Here's how the part is built. I have some questions about the finished solid (model axes, mm). Face numbers are marked on the shaded views. A direction names the side the tool comes from. Round coordinates to 2 decimals unless told otherwise and drop trailing zeros. Loops run counter-clockwise (first coordinate to the right, second up) from the corner with the lowest first, then second, coordinate; pieces in that order, holes last. Notation, with made-up numbers: M 29,-20.5 L 57,-20.5 A28 ccw 57,16.5 Z; hole C 79,4.5 d3. An arc over 180 degrees is marked long. Write each question's results on one line, items separated by ' | '. Start each with the question number.
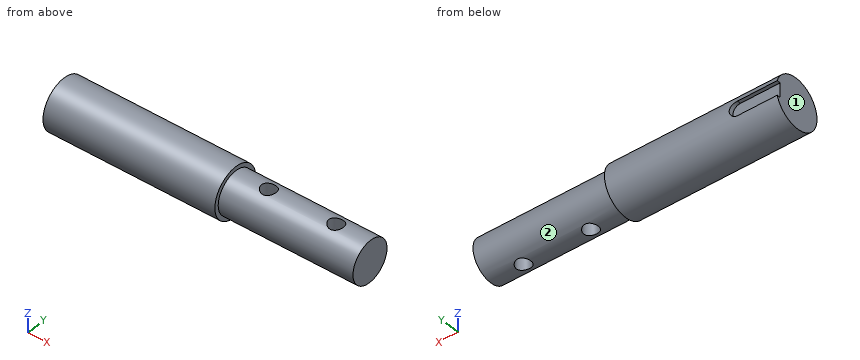
```python
from build123d import *

# Parameters (mm, degrees)
SKETCH1_R               = 37.5
BOSS_EXTRUDE1_DEPTH     = 255
SKETCH2_R               = 31.34
BOSS_EXTRUDE2_DEPTH     = 200
CUT_EXTRUDE1_DEPTH      = 7
CUT_EXTRUDE2_DEPTH      = 459.080233163
CUT_EXTRUDE2_DEPTH_BACK = 459.080233163
SKETCH4_R               = 11


with BuildPart() as part:
    # Sketch1 → Boss-Extrude1 (new body)
    with BuildSketch(Plane(origin=(0, 0, 0), x_dir=(0, 0, -1), z_dir=(1, 0, 0))):
        Circle(SKETCH1_R)
    extrude(amount=BOSS_EXTRUDE1_DEPTH)

    # Sketch2 → Boss-Extrude2 (add)
    with BuildSketch(Plane(origin=(255, 0, 0), x_dir=(0, 0, -1), z_dir=(1, 0, 0))):
        Circle(SKETCH2_R)
    extrude(amount=BOSS_EXTRUDE2_DEPTH)

    # Sketch3 → Cut-Extrude1 (cut)
    with BuildSketch(Plane(origin=(0, 37.5, 0), x_dir=(1, 0, 0), z_dir=(0, 1, 0))):
        with BuildLine():
            Line((59, -11), (0, -11))
            Line((0, -11), (0, 11))
            Line((0, 11), (59, 11))
            ThreePointArc((59, 11), (70, 0), (59, -11))
        make_face()
    extrude(amount=-CUT_EXTRUDE1_DEPTH, mode=Mode.SUBTRACT)

    # Sketch4 → Cut-Extrude2 (cut, two sides: drawn at the far end of the back side and taken through both)
    with BuildSketch(Plane.XY.offset(-CUT_EXTRUDE2_DEPTH_BACK)):
        with Locations((405, 0)):
            Circle(SKETCH4_R)
        with Locations((305, 0)):
            Circle(SKETCH4_R)
    extrude(amount=CUT_EXTRUDE2_DEPTH + CUT_EXTRUDE2_DEPTH_BACK, mode=Mode.SUBTRACT)


solid = part.part
```
1. I want a section at C-C on x = 98. List the corners of the cut face in (y, z) for me.
2. Which directions (+Z, -Z, +X, -X, +Y, -Y) give clear straight access to the entire face, cutting with the end or side of a thin tool? Please do the marked faces 1 and 2.
3. I need wall thicknesses on line 1 along X through (y, z) = (0, 9.5); line 2 along X through (y, z) = (-3, -27.5); line 3 along X through (y, z) = (16.5, -32). Which ranges of each line are inside material? Lowest first, please.
4. I want a section at D-D on x = 405. List the corners of the cut face in (y, z) for me.
5. I want a section at A-A on z = 0. List the corners of the cut face in (x, y) for me, plus the area to 3 significant figures.
6. I want a section at B-B on y = 0. List the corners of the cut face in (x, z) for me.
7. For pin 1 (4.5 mm diameter, centred on x = 18, y = 32, fed in from +Z); pin 2 (6 mm diameter, centred on x = 251.5, z = -15, fed in from -Y); pin 3 (5 mm diameter, centred on x = 366.5, y = 21.5, fed in from -Z), each with a flat end and sliding along its axis, tell me the tip position at first contact or that it passes through.
Outcome:
1) outline: C 0,0 d75
2) face 1: +Z, -Z, -X, +Y, -Y | face 2: +X
3) line 1: 0 to 294, 316 to 394, 416 to 455 | line 2: 0 to 294.42, 315.58 to 394.42, 415.58 to 455 | line 3: 0 to 255
4) outline: M -11,-29.35 L -11,29.35 A31.34 ccw Z; M 11,-29.35 A31.34 ccw 11,29.35 Z
5) outline: M 0,-37.5 L 255,-37.5 L 255,-31.34 L 455,-31.34 L 455,31.34 L 255,31.34 L 255,37.5 L 70,37.5 L 70,30.5 L 0,30.5 Z; hole C 305,0 d22; hole C 405,0 d22 | area: 30,400 mm2
6) outline: M 0,-37.5 L 255,-37.5 L 255,-31.34 L 294,-31.34 L 294,31.34 L 255,31.34 L 255,37.5 L 0,37.5 Z; M 316,-31.34 L 394,-31.34 L 394,31.34 L 316,31.34 Z; M 416,-31.34 L 455,-31.34 L 455,31.34 L 416,31.34 Z
7) pin 1: z = 22.83 | pin 2: y = -35.53 | pin 3: z = -24.92
